from build123d import *

# Parameters (mm, degrees)
SHELL1_T = -2.032


with BuildPart() as part:
    # Sketch1 → Revolve1 (revolve)
    with BuildSketch(Plane.XY):
        Polygon((0, 139.7), (59.6773, 139.7), (78.359, 38.1), (76.1619, 38.1), (76.1619, 0), (0, 0), align=None)
    revolve(axis=Axis((0, 0, 0), (0, 1, 0)))

    # Shell1
    shell1_openings = [part.faces().sort_by_distance(p)[0] for p in [
        (0, 0, 0),
        (0, 139.7, 0),
    ]]
    offset(amount=SHELL1_T, openings=shell1_openings, kind=Kind.INTERSECTION)


solid = part.part
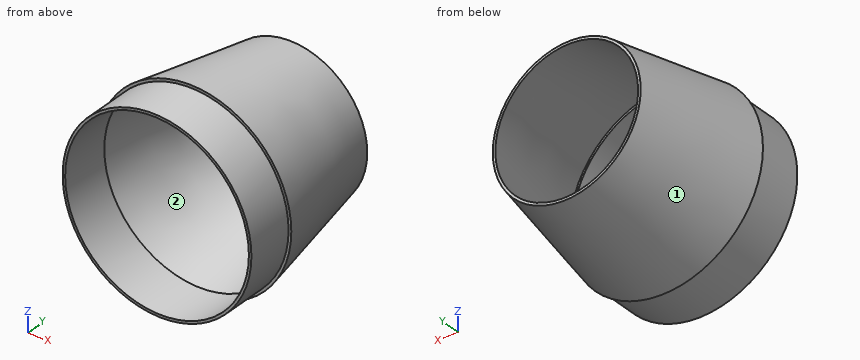
Geometry check sheet. Reference: the model listing, model coordinates, mm. Face numbers are marked on the shaded views. Give positions to 0.01 mm unless a question says otherwise; leave off trailing zeros. Order: outer loops, then holes, each group sorted by start corner. A loop starts at its lowest first (then second) coordinate and runs counter-clockwise, first axis right, second up. Notation, with made-up numbers: M 37.5,-32 L 92.5,-32 A22 cw 92.5,-5 Z; hole C 13.25,-23 d11. An arc over 180 degrees is marked long. Use a Markdown table: item, result.
Item 1: Material ranges on line 1 along Z through (x, y) = (0, 27.5); line 2 along X through (y, z) = (9, 36); line 3 along Z through (x, y) = (53, 132.5), recorded low to high.
Answers follow:
| item | result |
|---|---|
| line 1 | z = -76.16 to -74.13, 74.13 to 76.16 |
| line 2 | x = -67.12 to -64.8, 64.8 to 67.12 |
| line 3 | z = -30.2 to -25.77, 25.77 to 30.2 |
Item 2: Section check C-C (y = 22). Record the cut outline in (x, z).
Answers follow:
| item | result |
|---|---|
| outline | C 0,0 d152.32; hole C 0,0 d148.26 |
Item 3: Section check A-A (x = 0). Record the cut outline in (y, z), and give its area (3 significant figures).
Answers follow:
| item | result |
|---|---|
| outline | M 0,-76.16 L 38.1,-76.16 L 38.1,-78.36 L 139.7,-59.68 L 139.7,-57.61 L 40.13,-75.92 L 40.13,-74.13 L 0,-74.13 Z; M 0,74.13 L 40.13,74.13 L 40.13,75.92 L 139.7,57.61 L 139.7,59.68 L 38.1,78.36 L 38.1,76.16 L 0,76.16 Z |
| area | 583 mm2 |
Item 4: Depth check by flat-ended pin: P1, Ø5, axis at y = 64.5, z = 25.5, coming from the +X side; P2, Ø2, axis at x = 58, y = 57, coming from the -Z side; P3, Ø2, axis at y = 74.5, z = 49, coming from the -X side. Enter the tip coordinate at first touch or a pass-through.
Answers follow:
| item | result |
|---|---|
| P1 | stops at x = 69.94 |
| P2 | stops at z = -48.6 |
| P3 | stops at x = -53.25 |
Item 5: Draft check along X on the marked faces 1 and 2. Enter one of: +X half, -X half, draft (parallel to the pull), parting line (faces both ways), or undercut.
Answers follow:
| item | result |
|---|---|
| face 1 | parting line |
| face 2 | undercut |
Item 6: Section check B-B (z = 0). Record the cut outline in (x, y).
Answers follow:
| item | result |
|---|---|
| outline | M -78.36,38.1 L -76.16,38.1 L -76.16,0 L -74.13,0 L -74.13,40.13 L -75.92,40.13 L -57.61,139.7 L -59.68,139.7 Z; M 57.61,139.7 L 75.92,40.13 L 74.13,40.13 L 74.13,0 L 76.16,0 L 76.16,38.1 L 78.36,38.1 L 59.68,139.7 Z |
